```python
from build123d import *

# Parameters (mm, degrees)
BOSS_EXTRUDE1_DEPTH         = 158.750001
BOSS_EXTRUDE1_DEPTH_BACK    = 158.750001
SKETCH3_W                   = 50.8
SKETCH3_H                   = 25.4
SKETCH3_W_2                 = 47.625
SKETCH3_H_2                 = 22.225
SKETCH4_R                   = 14.2875
CUT_EXTRUDE1_DEPTH          = 39.37
F_10_CLEARANCE_HOLE1_D      = 4.9784
F_10_CLEARANCE_HOLE2_D      = 4.9784
F_20_0_161_DIAMETER_HOLE1_D = 4.0894
F_10_CLEARANCE_HOLE3_D      = 4.9784
F_10_CLEARANCE_HOLE3_DEPTH  = 12.7
F_10_CLEARANCE_HOLE3_TIP    = 1.495662253


with BuildPart() as part:
    # Sketch3 → Boss-Extrude1 (new, two sides: drawn at the far end of the back side and taken through both)
    with BuildSketch(Plane.XY.offset(-BOSS_EXTRUDE1_DEPTH_BACK)):
        Rectangle(SKETCH3_W, SKETCH3_H)
        Rectangle(SKETCH3_W_2, SKETCH3_H_2, mode=Mode.SUBTRACT)
    extrude(amount=BOSS_EXTRUDE1_DEPTH + BOSS_EXTRUDE1_DEPTH_BACK)

    # Sketch4 → Cut-Extrude1 (cut)
    with BuildSketch(Plane(origin=(0, 12.7, 0), x_dir=(1, 0, 0), z_dir=(0, 1, 0))):
        with Locations(Location((9.525, 95.250000508, 0), (0, 0, 180))):
            Circle(SKETCH4_R)
    extrude(amount=-CUT_EXTRUDE1_DEPTH, mode=Mode.SUBTRACT)

    # #10 Clearance Hole1 (through all)
    with Locations(Plane.ZY.offset(25.4)):
        with Locations((73.358188649, -2.425), (47.958188649, -2.425)):
            Hole(F_10_CLEARANCE_HOLE1_D / 2)

    # #10 Clearance Hole2 (through all)
    with Locations(Plane(origin=(0, -12.7, 0), x_dir=(-1, 0, 0), z_dir=(0, -1, 0))):
        with Locations((19.05, -51.113080493), (19.05, -89.213080493), (-19.05, -89.213080493), (-19.05, -152.400000508), (19.05, -152.400000508)):
            Hole(F_10_CLEARANCE_HOLE2_D / 2)

    # #20 (0.161) Diameter Hole1 (through all)
    with Locations(Plane(origin=(0, 12.7, 0), x_dir=(1, 0, 0), z_dir=(0, 1, 0))):
        with Locations((13.524629742, 112.574300261), (5.525370258, 77.925700755)):
            Hole(F_20_0_161_DIAMETER_HOLE1_D / 2)

    # #10 Clearance Hole3
    with Locations(Plane(origin=(25.4, 0, 0), x_dir=(0, 0, -1), z_dir=(1, 0, 0))):
        with Locations((-105.917999492, 0), (146.050000508, 0)):
            Hole(F_10_CLEARANCE_HOLE3_D / 2, depth=F_10_CLEARANCE_HOLE3_DEPTH)
            with Locations((0, 0, -(F_10_CLEARANCE_HOLE3_DEPTH + F_10_CLEARANCE_HOLE3_TIP / 2))):  # 118° drill point
                Cone(0, F_10_CLEARANCE_HOLE3_D / 2, F_10_CLEARANCE_HOLE3_TIP, mode=Mode.SUBTRACT)


solid = part.part
```
Build history of the part. All positions in model axes, mm. A direction names the side the tool comes from. Coordinates: 2 decimals unless noted, no trailing zeros. Write each loop counter-clockwise with the first axis right and the second up, starting at its lowest first coordinate (ties: lowest second). Pieces come first, ordered by that corner, then holes.
1. Drop a flat-ended pin along its axis: pin 1 (4 mm diameter, centred on x = -19.05, z = 89.21, fed in from +Y). Give the stop position or say it passes through.
Answer block:
pin 1: passes through
2. 3-axis set-ups, long thin cutter, end or side, ignore diameter. For faces 1 (the flat face through (23.812, 0, -2)), 2 (the cylindrical face through (24.595, 0.748, -143.676)), 3 (the cylindrical face through (-19.59, 11.917, 91.643)): which of +Z, -Z, +X, -X, +Y, -Y reach the whole face in a straight line?
Answer block:
face 1: +Z, -Z
face 2: +X
face 3: +Y, -Y
3. Drill centre lines: probe 1 along X at (y, z) = (-4.5, -38); probe 2 along X at (y, z) = (-12.3, -95.25); probe 3 along Y at (x, z) = (18.5, 52). Where is each one in solid material? Low to high.
Answer block:
probe 1: x = -25.4 to -23.81, 23.81 to 25.4
probe 2: x = -25.4 to -4.76, 23.81 to 25.4
probe 3: y = -12.7 to -11.11, 11.11 to 12.7
4. Band-saw the part on A-A, the plane z = 99. Give the cut face in (x, y), and give its area (3 significant figures).
Answer block:
outline: (-25.4, -12.7) - (25.4, -12.7) - (25.4, 12.7) - (-25.4, 12.7) - close; hole (-23.81, -11.11) - (23.81, -11.11) - (23.81, 11.11) - (-23.81, 11.11) - close
area: 232 mm2
5. Pull direction Y, two halves, no side cores. Call faces 4 (the cylindrical face through (-20.885, -11.895, 150.718)), 5 (the cylindrical face through (-24.595, -2.316, 50.445)), 6 (the flat face through (0, -12.7, -2)): released by +Y, released by -Y, zero draft, split by the parting line, or undercut.
Answer block:
face 4: zero draft
face 5: undercut
face 6: released by -Y
